Input: part model. Units: mm. Frame: model coordinates. Round coordinates to 2 decimals unless told otherwise and drop trailing zeros.
1) First-contact query: pin 1 (1.2 mm diameter, centred on y = 125, z = -2.5, fed in from +X). Flat tip, straight axial feed; report the tip coordinate or a pass-through.
2) Section A-A, the plane x = 165.5. State how many separate pieces and enclosed holes the cut face has, and give its area (3 significant figures).
3) Ray query, line 1 along Y through (x, z) = (224.5, -0.5); line 2 along Y through (x, z) = (188.5, -0.55); line 3 along Y through (x, z) = (160.5, -1.7). Return the intervals inside material, ascending.
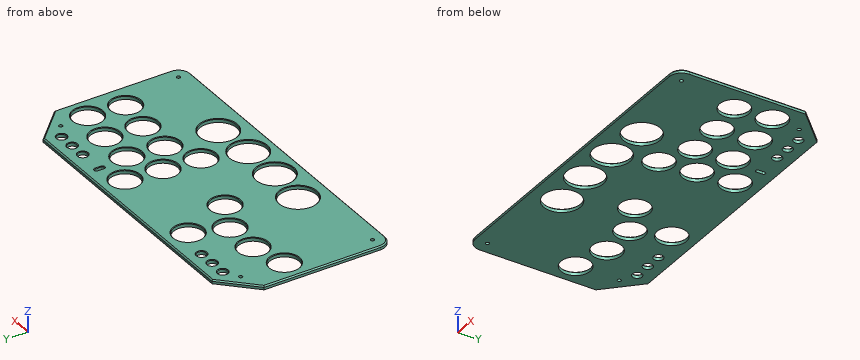
from build123d import *

# Parameters (mm, degrees)
BOSS_EXTRUDE1_DEPTH   = 3
SKETCH24_R            = 3.9
CUT_EXTRUDE2_DEPTH    = 307.167536128
SKETCH1_R             = 12
SKETCH1_R_2           = 15
CUT_EXTRUDE3_DEPTH    = 307.167536128
F_3_0MM_DOWEL_HOLE1_D = 3
CHAMFER1_SIZE         = 1
CHAMFER2_SIZE         = 0.5


with BuildPart() as part:
    # Sketch2 → Boss-Extrude1 (new body)
    with BuildSketch(Plane.XY):
        with BuildLine():
            Line((8.41186441, 15.286374556), (8.41186441, 109.410267401))
            Line((8.41186441, 109.410267401), (6.41186441, 107.410267401))
            Line((6.41186441, 107.410267401), (6.41186441, 15.286374556))
            ThreePointArc((6.41186441, 15.286374556), (9.340796598, 8.215306744), (16.41186441, 5.286374556))
            Line((16.41186441, 5.286374556), (264.168886442, 5.286374556))
            ThreePointArc((264.168886442, 5.286374556), (271.239954254, 8.215306744), (274.168886442, 15.286374556))
            Line((274.168886442, 15.286374556), (274.168886442, 107.410267401))
            Line((274.168886442, 107.410267401), (272.168886442, 109.410267401))
            Line((272.168886442, 109.410267401), (272.168886442, 15.286374556))
            ThreePointArc((272.168886442, 15.286374556), (269.825740692, 9.629520306), (264.168886442, 7.286374556))
            Line((264.168886442, 7.286374556), (16.41186441, 7.286374556))
            ThreePointArc((16.41186441, 7.286374556), (10.755010161, 9.629520306), (8.41186441, 15.286374556))
        make_face()
        with BuildLine():
            Line((247.340459317, 134.238694526), (33.240291535, 134.238694526))
            Line((33.240291535, 134.238694526), (8.41186441, 109.410267401))
            Line((8.41186441, 109.410267401), (8.41186441, 15.286374556))
            ThreePointArc((8.41186441, 15.286374556), (10.755010161, 9.629520306), (16.41186441, 7.286374556))
            Line((16.41186441, 7.286374556), (264.168886442, 7.286374556))
            ThreePointArc((264.168886442, 7.286374556), (269.825740692, 9.629520306), (272.168886442, 15.286374556))
            Line((272.168886442, 15.286374556), (272.168886442, 109.410267401))
            Line((272.168886442, 109.410267401), (247.340459317, 134.238694526))
        make_face()
        Polygon((33.240291535, 134.238694526), (30.41186441, 134.238694526), (8.41186441, 112.238694526), (8.41186441, 109.410267401), align=None)
        Polygon((8.41186441, 109.410267401), (8.41186441, 112.238694526), (6.41186441, 110.238694526), (6.41186441, 107.410267401), align=None)
        Polygon((32.41186441, 136.238694526), (30.41186441, 134.238694526), (33.240291535, 134.238694526), (35.240291535, 136.238694526), align=None)
        Polygon((35.240291535, 136.238694526), (33.240291535, 134.238694526), (247.340459317, 134.238694526), (245.340459317, 136.238694526), align=None)
        Polygon((272.168886442, 112.238694526), (272.168886442, 109.410267401), (274.168886442, 107.410267401), (274.168886442, 110.238694526), align=None)
        Polygon((250.168886442, 134.238694526), (247.340459317, 134.238694526), (272.168886442, 109.410267401), (272.168886442, 112.238694526), align=None)
        Polygon((245.340459317, 136.238694526), (247.340459317, 134.238694526), (250.168886442, 134.238694526), (248.168886442, 136.238694526), align=None)
    extrude(amount=-BOSS_EXTRUDE1_DEPTH)

    # Sketch24 → Cut-Extrude2 (cut, through all)
    with BuildSketch(Plane.XY):
        with Locations((37.41186441, 124.238694526)):
            Circle(SKETCH24_R)
        with Locations((50.91186441, 124.238694526)):
            Circle(SKETCH24_R)
        with Locations((64.41186441, 124.238694526)):
            Circle(SKETCH24_R)
        with Locations((216.168886442, 124.238694526)):
            Circle(SKETCH24_R)
        with Locations((229.668886442, 124.238694526)):
            Circle(SKETCH24_R)
        with Locations((243.168886442, 124.238694526)):
            Circle(SKETCH24_R)
        with BuildLine():
            Line((193.298949614, 126.738694526), (193.298949614, 121.738694526))
            ThreePointArc((193.298949614, 121.738694526), (194.798949614, 120.238694526), (196.298949614, 121.738694526))
            Line((196.298949614, 121.738694526), (196.298949614, 126.738694526))
            ThreePointArc((196.298949614, 126.738694526), (194.798949614, 128.238694526), (193.298949614, 126.738694526))
        make_face()
    extrude(amount=-CUT_EXTRUDE2_DEPTH, mode=Mode.SUBTRACT)

    # Sketch1 → Cut-Extrude3 (cut, through all)
    with BuildSketch(Plane.XY):
        with Locations((24.41186441, 82.179064133)):
            Circle(SKETCH1_R)
        with Locations((52.996556322, 89.470524089)):
            Circle(SKETCH1_R)
        with Locations((92.45540719, 117.238694526)):
            Circle(SKETCH1_R)
        with Locations((82.496556322, 89.470524089)):
            Circle(SKETCH1_R)
        with Locations((109.001946024, 76.520067852)):
            Circle(SKETCH1_R)
        with Locations((168.091946024, 58.360067852)):
            Circle(SKETCH1_R)
        with Locations((194.873540874, 70.729230202)):
            Circle(SKETCH1_R)
        with Locations((224.358659158, 69.792320505)):
            Circle(SKETCH1_R)
        with Locations((253.510608286, 65.274150291)):
            Circle(SKETCH1_R)
        with Locations((256.168886442, 94.654135948)):
            Circle(SKETCH1_R)
        with Locations((227.016937315, 99.172306162)):
            Circle(SKETCH1_R)
        with Locations((197.531819031, 100.10921586)):
            Circle(SKETCH1_R)
        with Locations((170.75022418, 87.740053509)):
            Circle(SKETCH1_R)
        with Locations((191.774681199, 29.091460603)):
            Circle(SKETCH1_R_2)
        with Locations((157.891946024, 26.270067852)):
            Circle(SKETCH1_R_2)
        with Locations((123.891946024, 26.270067852)):
            Circle(SKETCH1_R_2)
        with Locations((90.009210849, 29.091460603)):
            Circle(SKETCH1_R_2)
        with Locations((173.429012786, 117.118176179)):
            Circle(SKETCH1_R)
    extrude(amount=-CUT_EXTRUDE3_DEPTH, mode=Mode.SUBTRACT)

    # 3.0mm Dowel Hole1 (through all)
    with Locations(Plane.XY):
        with Locations((25.42227205, 117.228286886), (16.41186441, 15.286374556), (264.168886442, 15.286374556), (255.158478802, 117.228286886)):
            Hole(F_3_0MM_DOWEL_HOLE1_D / 2)

    # Chamfer1
    chamfer1_edges = [part.edges().sort_by_distance(p)[0] for p in [
        (274.168886442, 62.762534541, 0),
        (271.239954254, 8.215306744, 0),
        (140.290375426, 5.286374556, 0),
        (9.340796598, 8.215306744, 0),
        (6.41186441, 62.762534541, 0),
        (19.41186441, 123.238694526, 0),
        (140.290375426, 136.238694526, 0),
        (261.168886442, 123.238694526, 0),
    ]]
    chamfer(chamfer1_edges, length=CHAMFER1_SIZE)

    # Chamfer2
    chamfer2_edges = [part.edges().sort_by_distance(p)[0] for p in [
        (12.41186441, 82.179064133, 0),
        (161.429012786, 117.118176179, 0),
        (97.001946024, 76.520067852, 0),
        (80.45540719, 117.238694526, 0),
        (70.496556322, 89.470524089, 0),
        (40.996556322, 89.470524089, 0),
        (75.009210849, 29.091460603, 0),
        (108.891946024, 26.270067852, 0),
        (142.891946024, 26.270067852, 0),
        (176.774681199, 29.091460603, 0),
        (158.75022418, 87.740053509, 0),
        (185.531819031, 100.10921586, 0),
        (215.016937315, 99.172306162, 0),
        (244.168886442, 94.654135948, 0),
        (241.510608286, 65.274150291, 0),
        (212.358659158, 69.792320505, 0),
        (182.873540874, 70.729230202, 0),
        (156.091946024, 58.360067852, 0),
        (33.51186441, 124.238694526, 0),
        (194.798949614, 128.238694526, 0),
        (193.298949614, 124.238694526, 0),
        (194.798949614, 120.238694526, 0),
        (196.298949614, 124.238694526, 0),
        (239.268886442, 124.238694526, 0),
        (225.768886442, 124.238694526, 0),
        (212.268886442, 124.238694526, 0),
        (60.51186441, 124.238694526, 0),
        (47.01186441, 124.238694526, 0),
    ]]
    chamfer(chamfer2_edges, length=CHAMFER2_SIZE)


solid = part.part
Final values:
1. pin 1: stops at x = 260.01
2. separate pieces: 5
2. enclosed holes: 0
2. area: 124 mm2
3. line 1: y = 5.79 to 57.79, 81.79 to 87.44, 110.91 to 135.74
3. line 2: y = 5.74 to 14.45, 43.73 to 60.56, 80.9 to 92.21, 108.01 to 135.79
3. line 3: y = 5.29 to 11.5, 41.04 to 49.07, 67.65 to 81.5, 93.98 to 136.24
